```python
from build123d import *

# Parameters (mm, degrees)
BOSS_EXTRUDE1_DEPTH = 146.05
SKETCH2_W           = 63.5
SKETCH2_H           = 76.2
CUT_EXTRUDE1_DEPTH  = 146.05
BOSS_EXTRUDE2_DEPTH = 12.7
SKETCH4_R           = 6.35
CUT_EXTRUDE2_DEPTH  = 12.7


with BuildPart() as part:
    # Sketch1 → Boss-Extrude1 (new body)
    with BuildSketch(Plane(origin=(0, 0, 0), x_dir=(0, 0, -1), z_dir=(1, 0, 0))):
        Polygon((0, 0), (-101.6, 0), (-101.6, 6.35), (-101.6, 234.95), (-95.25, 234.95), (-95.25, 6.35), (0, 6.35), align=None)
    extrude(amount=BOSS_EXTRUDE1_DEPTH)

    # Sketch2 → Cut-Extrude1 (cut)
    with BuildSketch(Plane.XY.offset(101.6)):
        with Locations((31.75, 38.1)):
            Rectangle(SKETCH2_W, SKETCH2_H)
    extrude(amount=-CUT_EXTRUDE1_DEPTH, mode=Mode.SUBTRACT)

    # Sketch3 → Boss-Extrude2 (add)
    with BuildSketch(Plane.ZY.offset(-63.5)):
        Polygon((0, 6.35), (95.25, 76.2), (95.25, 6.35), align=None)
    extrude(amount=-BOSS_EXTRUDE2_DEPTH)

    # Sketch4 → Cut-Extrude2 (cut)
    with BuildSketch(Plane(origin=(0, 6.35, 0), x_dir=(1, 0, 0), z_dir=(0, 1, 0))):
        with Locations(Location((111.125, -19.05, 0), (0, 0, 270))):
            Circle(SKETCH4_R)
        with Locations(Location((111.125, -82.55, 0), (0, 0, 270))):
            Circle(SKETCH4_R)
    extrude(amount=-CUT_EXTRUDE2_DEPTH, mode=Mode.SUBTRACT)


solid = part.part
```
Design review of the part built by this model. Coordinates are the model's own, in mm. A direction names the side the tool comes from. Coordinates: 2 decimals unless noted, no trailing zeros. Order: outer loops, then holes, each group sorted by start corner. A loop starts at its lowest first (then second) coordinate and runs counter-clockwise, first axis right, second up. Notation, with made-up numbers: (77, -18) - (130, -18) arc R30 ccw to (130, 8) - close; hole circle Ø4 at (36, 21). An arc over 180 degrees is marked (long way). Answer in a Markdown table with one row per item.
(1) Clearance check with flat-ended pins moving along their axes: pin 1 (5 mm diameter, centred on x = 18.5, z = 98.5, fed in from -Y); pin 2 (7.5 mm diameter, centred on x = 111.125, z = 82.55, fed in from +Y); pin 3 (10 mm diameter, centred on y = 23.5, z = 86.5, fed in from +X); pin 4 (3 mm diameter, centred on x = 48.5, y = 145, fed in from -Z). State where each tip first meets the part, or that it passes through.
Checked values:
| item | result |
|---|---|
| pin 1 | y = 76.2 |
| pin 2 | through |
| pin 3 | x = 76.2 |
| pin 4 | z = 95.25 |
(2) Wall thickness on line 1 along X through (y, z) = (5, 19); line 2 along Z through (x, y) = (21.5, 154); line 3 along Y through (x, z) = (92.5, 10): over which ranges is each line inside the solid? List them lowest first. Write a range as from..to.
Checked values:
| item | result |
|---|---|
| line 1 | 63.5..104.78, 117.47..146.05 |
| line 2 | 95.25..101.6 |
| line 3 | 0..6.35 |
(3) For faces 1 (the flat face through (31, 76.2, 98)), 2 (the flat face through (76.2, 26, 69)), 3 (the flat face through (146.05, 83, 96)), list the 3-axis set-ups (+Z, -Z, +X, -X, +Y, -Y) from which the entire face can be reached by the end or side of a thin tool; tool diameter is ignored.
Checked values:
| item | result |
|---|---|
| face 1 | +Z, -Z, -X, -Y |
| face 2 | -Z, +X, +Y |
| face 3 | +Z, -Z, +X, +Y, -Y |
(4) Consider section C-C on y = 175. State the section outline as (x, z) points.
Checked values:
| item | result |
|---|---|
| outline | (0, 95.25) - (146.05, 95.25) - (146.05, 101.6) - (0, 101.6) - close |
(5) The part is to be moulded in two halves that separate along Z. For faces 4 (the cylindrical face through (104.926, 3.219, 81.173)), 5 (the flat face through (72, 148, 95.25)), 6 (the flat face through (104, 0, 50)), say which applies: released by +Z, released by -Z, zero draft, split by the parting line, or undercut.
Checked values:
| item | result |
|---|---|
| face 4 | undercut |
| face 5 | released by -Z |
| face 6 | zero draft |
(6) Consider section D-D on z = 56.5. State the section outline as (x, y) points.
Checked values:
| item | result |
|---|---|
| outline | (63.5, 0) - (146.05, 0) - (146.05, 6.35) - (76.2, 6.35) - (76.2, 47.78) - (63.5, 47.78) - close |
(7) Consider section B-B on x = 73. State the section outline as (y, z) points.
Checked values:
| item | result |
|---|---|
| outline | (0, 0) - (6.35, 0) - (76.2, 95.25) - (234.95, 95.25) - (234.95, 101.6) - (0, 101.6) - close |
(8) Consider section A-A on z = 19.05. State the section outline as (x, y) points (3 decimals), plus the area to 3 significant figures.
Checked values:
| item | result |
|---|---|
| outline | (63.5, 0) - (104.775, 0) - (104.775, 6.35) - (76.2, 6.35) - (76.2, 20.32) - (63.5, 20.32) - close; (117.475, 0) - (146.05, 0) - (146.05, 6.35) - (117.475, 6.35) - close |
| area | 621 mm^2 |
